The listing builds one solid part. Answer for the finished solid, in the listing's coordinates (mm). Face numbers are marked on the shaded views. A direction names the side the tool comes from. Give positions to 0.01 mm unless a question says otherwise; leave off trailing zeros. Order: outer loops, then holes, each group sorted by start corner. A loop starts at its lowest first (then second) coordinate and runs counter-clockwise, first axis right, second up.
Autodesk Inventor part; units mm, degrees
ref_plane "Work Plane4" through (0, 0, 0) normal (0, -1, 0) x (1, 0, 0)
ref_plane "Work Plane2" through (0, 0, 0) normal (0, -1, 0) x (1, 0, 0)
ref_plane "Work Plane5" through (0, 1.6, 0) normal (0, 1, 0) x (1, 0, 0)
ref_plane "Work Plane4" through (0, 0, 0) normal (0, -1, 0) x (1, 0, 0)
sketch "Sketch2" plane through (0, 0, 0) normal (0, -1, 0) x (1, 0, 0)
  circle A0 centre (0, 0) radius 1.9
  dimension "d34" = 3.8
extrude "Extrusion4" add sketch "Sketch2" against normal blind 1.3
ref_plane "Work Plane2" through (0, 0, 0) normal (0, -1, 0) x (1, 0, 0)
sketch "Sketch4" plane through (0, 0, 0) normal (0, -1, 0) x (1, 0, 0)
  arc A0 (-0.25, -1.8835) -> (0.25, -1.8835) centre (0, 0) ccw
  arc A1 (0.25, 1.8835) -> (-0.25, 1.8835) centre (0, 0) ccw
  line L0 (0.25, 0.25) -> (1.8835, 0.25)
  line L1 (-0.25, 0.25) -> (-1.8835, 0.25)
  arc A2 (-0.25, -1.8835) -> (0.25, -1.8835) centre (0, 0) ccw
  arc A3 (1.8835, -0.25) -> (1.8835, 0.25) centre (0, 0) ccw
  arc A4 (0.25, 1.8835) -> (-0.25, 1.8835) centre (0, 0) ccw
  arc A5 (-1.8835, 0.25) -> (-1.8835, -0.25) centre (0, 0) ccw
  line L2 (1.8835, -0.25) -> (0.25, -0.25)
  line L3 (-0.25, -0.25) -> (-1.8835, -0.25)
  line L4 (-0.25, -1.8835) -> (-0.25, -0.25)
  line L5 (-0.25, 0.25) -> (-0.25, 1.8835)
  line L6 (0.25, -1.8835) -> (0.25, -0.25)
  line L7 (0.25, 0.25) -> (0.25, 1.8835)
extrude "Extrusion5" cut sketch "Sketch4" against normal blind 0.4
ref_plane "Work Plane5" through (0, 1.6, 0) normal (0, 1, 0) x (1, 0, 0)
ref_plane "Work Plane6" through (0, 1.3, 0) normal (0, 1, 0) x (1, 0, 0)
sketch "Sketch6" plane through (0, 1.3, 0) normal (0, 1, 0) x (1, 0, 0)
  circle A0 centre (0, 0) radius 1
  dimension "d35" = 2
extrude "Extrusion7" add sketch "Sketch6" along normal blind 5
thread "Thread4"
properties part number "M2x6_D963"
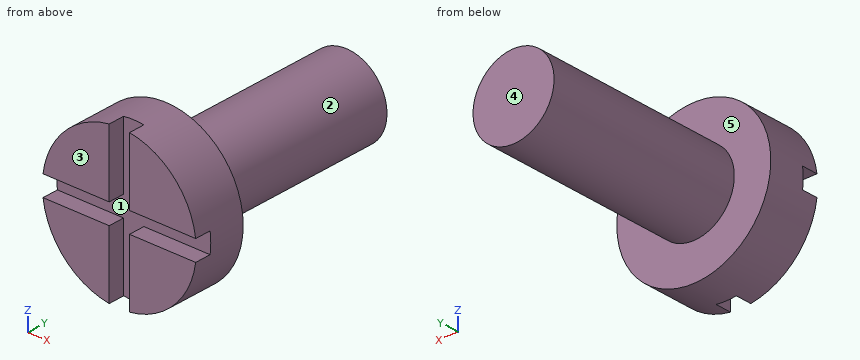
1) Find section B-B (x = 0). Write down the section's boundary in (y, z).
Geometry says:
outline: (0.4, -1.9) - (1.3, -1.9) - (1.3, -1) - (6.3, -1) - (6.3, 1) - (1.3, 1) - (1.3, 1.9) - (0.4, 1.9) - close
2) Find section C-C (y = 5.75). Write down the section's boundary in (x, z), then the cut area to 3 significant figures.
Geometry says:
outline: circle Ø2 at (0, 0)
area: 3.14 mm2
3) Find section A-A (z = 0). Write down the section's boundary in (x, y), then the cut area to 3 significant figures.
Geometry says:
outline: (-1.9, 0.4) - (1.9, 0.4) - (1.9, 1.3) - (1, 1.3) - (1, 6.3) - (-1, 6.3) - (-1, 1.3) - (-1.9, 1.3) - close
area: 13.4 mm2
4) Straight lines are drawn through the part: probe 1 along Y at (x, z) = (-1.2, -0.85); probe 2 along Y at (x, z) = (0.1, 1.15); probe 3 along X at (y, z) = (0.5, 0.5). For each, find the intervals that lie inside material, in ascending order.
Geometry says:
probe 1: y = 0 to 1.3
probe 2: y = 0.4 to 1.3
probe 3: x = -1.83 to 1.83
5) Find section D-D (z = 0.85). Write down the section's boundary in (x, y).
Geometry says:
outline: (-1.7, 0) - (-0.25, 0) - (-0.25, 0.4) - (0.25, 0.4) - (0.25, 0) - (1.7, 0) - (1.7, 1.3) - (0.53, 1.3) - (0.53, 6.3) - (-0.53, 6.3) - (-0.53, 1.3) - (-1.7, 1.3) - close
6) For a pull along Z with two mould halves and no side action, classify the marked faces 1, 2 and 3 as +Z half, -Z half, draft (parallel to the pull), parting line (faces both ways), or undercut.
Geometry says:
face 1: undercut
face 2: parting line
face 3: draft
7) A tool of negligible diameter and unlimited length cuts with its end or side. For the marked faces 4 and 5, from which of +Z, -Z, +X, -X, +Y, -Y can it reach the whole face along a straight path? Write none if from no direction.
Geometry says:
face 4: +Z, -Z, +X, -X, +Y
face 5: +Y
